Here's the drawing with two shaded views (mm, measured from the low corner). I have some questions. Round coordinates to 2 decimals unless told otherwise and drop trailing zeros. Order: outer loops, then holes, each group sorted by start corner. A loop starts at its lowest first (then second) coordinate and runs counter-clockwise, first axis right, second up.
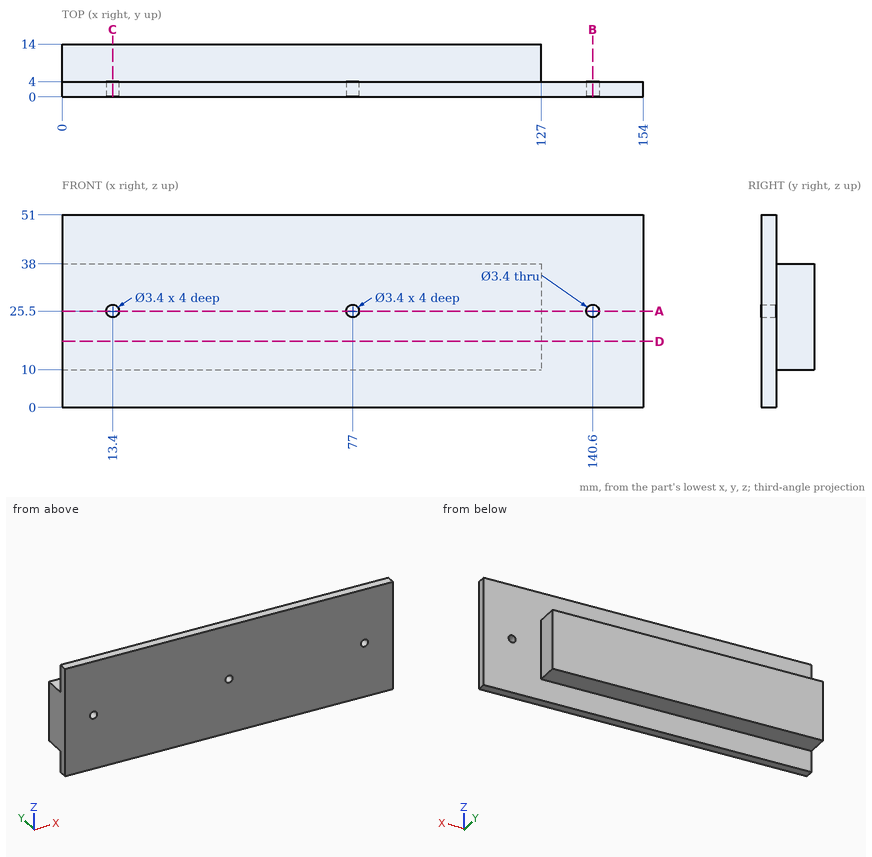
Q1. Imagine slicing it at B-B, the plane x = 140.6. Please give me the cut outline in (y, z), then the cut area to 3 significant figures.
Q2. I need wall thicknesses on L1, parallel to X at y = 3, z = 25.5; L2, parallel to Z at x = 140.6, y = 1.25; L3, parallel to Y at x = 57, z = 48. Which ranges of each line are inside material? Lowest first, please.
Q3. Imagine slicing it at C-C, the plane x = 13.4. Please give me the cut outline in (y, z).
Q4. For P1, Ø8, axis at x = 63.5, y = 10, coming from the +Z side; P2, Ø5, axis at x = 84.5, y = 7.5, coming from the -Z side; P3, Ø1.5, axis at y = 12.5, z = 8, coming from the +X side; P4, Ø2.5, axis at x = 77, z = 25.5, coming from the -Y side, each with a flat end and sliding along its axis, tell me the tip position at first contact or that it passes through.
Q5. Imagine slicing it at A-A, the plane z = 25.5. Please give me the cut outline in (x, y), then the cut area to 3 significant figures.
Q6. Imagine slicing it at D-D, the plane z = 17.5. Please give me the cut outline in (x, y), then the cut area to 3 significant figures.
Filled in:
1. outline: (0, 0) - (4, 0) - (4, 23.8) - (0, 23.8) - close; (0, 27.2) - (4, 27.2) - (4, 51) - (0, 51) - close
1. area: 190 mm2
2. L1: x = 0 to 11.7, 15.1 to 75.3, 78.7 to 138.9, 142.3 to 154
2. L2: z = 0 to 23.8, 27.2 to 51
2. L3: y = 0 to 4
3. outline: (0, 0) - (4, 0) - (4, 10) - (14, 10) - (14, 38) - (4, 38) - (4, 51) - (0, 51) - (0, 27.2) - (4, 27.2) - (4, 23.8) - (0, 23.8) - close
4. P1: stops at z = 38
4. P2: stops at z = 10
4. P3: passes through
4. P4: stops at y = 4
5. outline: (0, 0) - (11.7, 0) - (11.7, 4) - (15.1, 4) - (15.1, 0) - (75.3, 0) - (75.3, 4) - (78.7, 4) - (78.7, 0) - (138.9, 0) - (138.9, 4) - (127, 4) - (127, 14) - (0, 14) - close; (142.3, 0) - (154, 0) - (154, 4) - (142.3, 4) - close
5. area: 1,850 mm2
6. outline: (0, 0) - (154, 0) - (154, 4) - (127, 4) - (127, 14) - (0, 14) - close
6. area: 1,890 mm2
